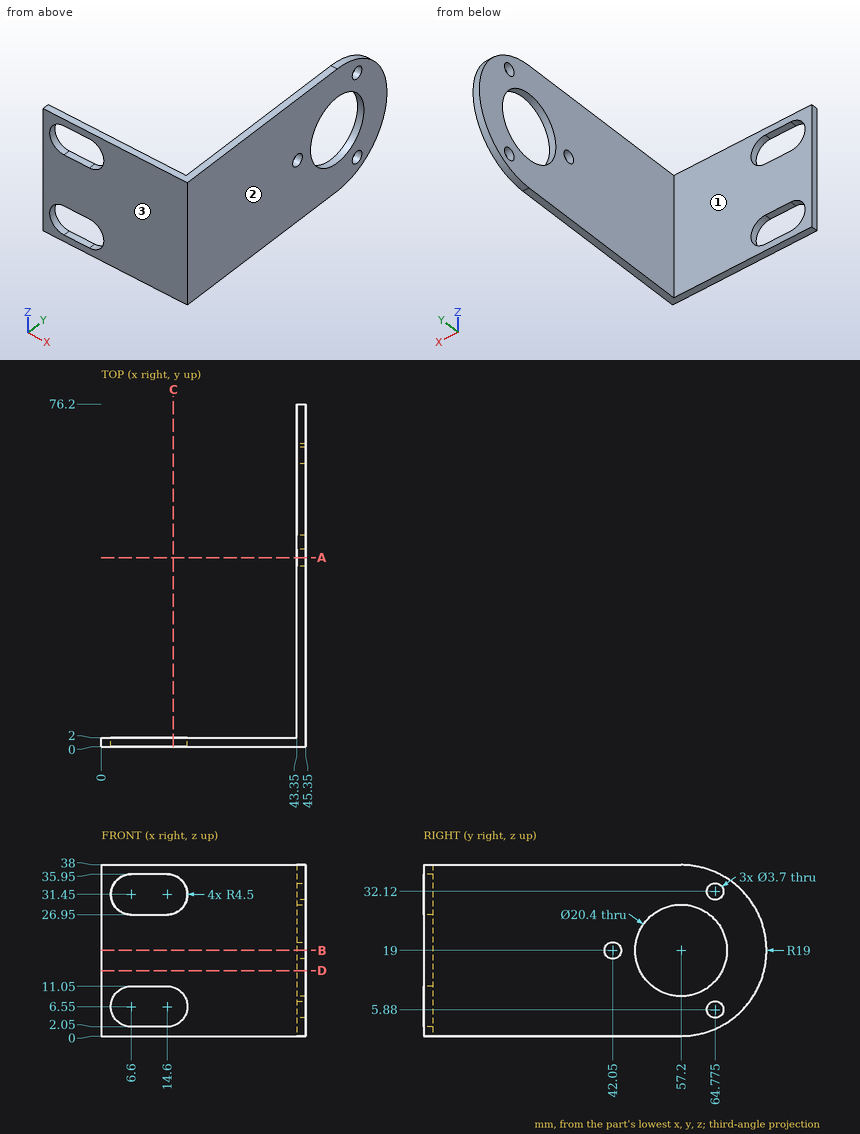
Study the drawing (mm; zero at the part's minimum x, y, z) and answer. Round coordinates to 2 decimals unless told otherwise and drop trailing zeros. Loops run counter-clockwise (first coordinate to the right, second up) from the corner with the lowest first, then second, coordinate; pieces in that order, holes last. Notation, with made-up numbers: (62.5, -22.5) -> (99.5, -22.5) arc R19 ccw to (99.5, 1.5) -> close; hole circle Ø2 at (57, 17.5). An arc over 180 degrees is marked (long way). Write each question's results on one line, items separated by ' | '. Start each with the question number.
1. Section A-A (y = 42.05) is taken. Determine the outline of the cut face in (x, z), plus the area to 3 significant figures.
2. For a pull along Y with two mould halves and no side action, classify the marked faces 1, 2 and 3 as +Y half, -Y half, draft (parallel to the pull), parting line (faces both ways), or undercut.
3. Section B-B (z = 19) is taken. Determine the outline of the cut face in (x, y), plus the area to 3 significant figures.
4. Find the intervals of material crossed by probe 1 along Y at (x, z) = (44.2, 19); probe 2 along Y at (x, z) = (43, 19); probe 3 along X at (y, z) = (18.5, 4.5), in increasing order. Write a range as from..to.
5. Section D-D (z = 14.5) is taken. Determine the outline of the cut face in (x, y).
6. Section C-C (x = 16) is taken. Determine the outline of the cut face in (y, z), plus the area to 3 significant figures.
7. Given pin 1 Ø3 at (x, z) = (31, 21.5) entering from +Y; pin 2 Ø1 at (y, z) = (34, 14) entering from -X; pin 3 Ø6 at (x, z) = (40.5, 22.5) entering from +Y, each flat-ended and moving along its own axis, determine where each tip first touches the part or whether it passes through.
Evaluation:
1) outline: (43.35, 0) -> (45.35, 0) -> (45.35, 17.15) -> (43.35, 17.15) -> close; (43.35, 20.85) -> (45.35, 20.85) -> (45.35, 38) -> (43.35, 38) -> close | area: 68.6 mm2
2) face 1: +Y half | face 2: draft | face 3: -Y half
3) outline: (0, 0) -> (45.35, 0) -> (45.35, 40.2) -> (43.35, 40.2) -> (43.35, 2) -> (0, 2) -> close; (43.35, 43.9) -> (45.35, 43.9) -> (45.35, 47) -> (43.35, 47) -> close; (43.35, 67.4) -> (45.35, 67.4) -> (45.35, 76.2) -> (43.35, 76.2) -> close | area: 191 mm2
4) probe 1: y = 0..40.2, 43.9..47, 67.4..76.2 | probe 2: y = 0..2 | probe 3: x = 43.35..45.35
5) outline: (0, 0) -> (45.35, 0) -> (45.35, 48.05) -> (43.35, 48.05) -> (43.35, 2) -> (0, 2) -> close; (43.35, 66.35) -> (45.35, 66.35) -> (45.35, 75.66) -> (43.35, 75.66) -> close
6) outline: (0, 0) -> (2, 0) -> (2, 2.27) -> (0, 2.27) -> close; (0, 10.83) -> (2, 10.83) -> (2, 27.17) -> (0, 27.17) -> close; (0, 35.73) -> (2, 35.73) -> (2, 38) -> (0, 38) -> close | area: 41.8 mm2
7) pin 1: stops at y = 2 | pin 2: stops at x = 43.35 | pin 3: stops at y = 76.03
